Input: part model. Units: mm. Frame: model coordinates. A direction names the side the tool comes from. Round coordinates to 2 decimals unless told otherwise and drop trailing zeros. Order: outer loops, then holes, each group sorted by start corner. A loop starts at its lowest first (then second) coordinate and runs counter-clockwise, first axis right, second up. Notation, with made-up numbers: (56, 86) - (113, 86) arc R21 ccw to (113, 120) - close; hole circle Ø5 at (38.5, 10.5). An arc over 180 degrees is marked (long way). One line per item, written item: value. Start each with the question number.
from build123d import *

# Parameters (mm, degrees)
BOSS_EXTRUDE6_DEPTH  = 2.05994
SKETCH9_W            = 27.13228
SKETCH9_H            = 1.41224
BOSS_EXTRUDE7_DEPTH  = 20.32
SKETCH10_R           = 2.50063
CUT_EXTRUDE3_DEPTH   = 25.4
BOSS_EXTRUDE10_DEPTH = 16.02994
SKETCH15_W           = 51.72964
SKETCH15_H           = 37.846
CUT_EXTRUDE5_DEPTH   = 64.999044225
SKETCH16_W           = 27.13228
SKETCH16_H           = 1.41224
BOSS_EXTRUDE11_DEPTH = 3.175
SKETCH18_W           = 12.7
SKETCH18_H           = 2.54
BOSS_EXTRUDE12_DEPTH = 12.7
SKETCH19_R           = 2.159
CUT_EXTRUDE6_DEPTH   = 62.075806811


with BuildPart() as part:
    # Sketch8 → Boss-Extrude6 (new body)
    with BuildSketch(Plane(origin=(0, 0, 0), x_dir=(1, 0, 0), z_dir=(0, 1, 0))):
        Polygon((-44.974060072, -2.900891689), (-44.974060072, -40.746891689), (2.165799928, -40.746891689), (2.165799928, -35.808024144), (6.755579928, -31.218244144), (33.887859928, -31.218244144), (33.887859928, -12.429539234), (6.755579928, -12.429539234), (2.165799928, -7.839759234), (2.165799928, -2.900891689), align=None)
    extrude(amount=BOSS_EXTRUDE6_DEPTH)

    # Sketch9 → Boss-Extrude7 (add)
    with BuildSketch(Plane(origin=(0, 2.05994, 0), x_dir=(1, 0, 0), z_dir=(0, 1, 0))):
        with Locations((20.321719928, -13.135659234)):
            Rectangle(SKETCH9_W, SKETCH9_H)
        with Locations((20.321719928, -30.512124144)):
            Rectangle(SKETCH9_W, SKETCH9_H)
    extrude(amount=BOSS_EXTRUDE7_DEPTH)

    # Sketch10 → Cut-Extrude3 (cut)
    with BuildSketch(Plane.XY.offset(31.218244144)):
        with Locations((29.955939928, 17.2847)):
            Circle(SKETCH10_R)
    extrude(amount=-CUT_EXTRUDE3_DEPTH, mode=Mode.SUBTRACT)

    # Sketch14 → Boss-Extrude10 (add)
    with BuildSketch(Plane.XY.offset(13.841779234)):
        Polygon((6.755579928, 22.37994), (33.887859928, 2.05994), (30.568919609, 2.05994), (6.755579928, 19.826826768), align=None)
    extrude(amount=BOSS_EXTRUDE10_DEPTH)

    # Sketch15 → Cut-Extrude5 (cut, through all)
    with BuildSketch(Plane(origin=(0, 2.05994, 0), x_dir=(1, 0, 0), z_dir=(0, 1, 0))):
        with Locations((-19.109240072, -21.823891689)):
            Rectangle(SKETCH15_W, SKETCH15_H)
    extrude(amount=-CUT_EXTRUDE5_DEPTH, mode=Mode.SUBTRACT)

    # Sketch16 → Boss-Extrude11 (add)
    with BuildSketch(Plane(origin=(0, 22.37994, 0), x_dir=(1, 0, 0), z_dir=(0, 1, 0))):
        with Locations((20.321719928, -30.512124144)):
            Rectangle(SKETCH16_W, SKETCH16_H)
        with Locations((20.321719928, -13.135659234)):
            Rectangle(SKETCH16_W, SKETCH16_H)
    extrude(amount=BOSS_EXTRUDE11_DEPTH)

    # Sketch18 → Boss-Extrude12 (add)
    with BuildSketch(Plane.XY.offset(31.218244144)):
        with Locations((13.105579928, 24.28494)):
            Rectangle(SKETCH18_W, SKETCH18_H)
    boss_extrude12 = extrude(amount=BOSS_EXTRUDE12_DEPTH)

    # Mirror1: Boss-Extrude12 across plane
    add(boss_extrude12.mirror(Plane.XY.offset(21.823891689)))

    # Sketch19 → Cut-Extrude6 (cut, through all)
    with BuildSketch(Plane(origin=(0, 25.55494, 0), x_dir=(1, 0, 0), z_dir=(0, 1, 0))):
        with Locations(Location((13.105579928, -6.079539234, 0), (0, 0, 270))):
            Circle(SKETCH19_R)
        with Locations(Location((13.105579928, -37.568244144, 0), (0, 0, 270))):
            Circle(SKETCH19_R)
    extrude(amount=-CUT_EXTRUDE6_DEPTH, mode=Mode.SUBTRACT)


solid = part.part
1. Section B-B (x = 20.5). Return the cut outline in (y, z), then the cut area to 3 significant figures.
2. Section D-D (y = 10.5). Return the cut outline in (x, z).
3. Set-up query: faces 1 (the face through (16, 23.015, 6)), 2 (the face through (18, 2.06, 22)), 3 (the face through (19.456, 24, 37)), 4 (the face through (23, 19, 29.806)), 5 (the face through (13, 24, 43.918)). Return all of +Z, -Z, +X, -X, +Y, -Y with unobstructed straight access to the full face (end or side cutting, diameter ignored); none if empty.
4. Section A-A (x = 14.25). Return the cut outline in (y, z).
5. Pin query (flat end, axial travel): pin 1 (11.5 mm diameter, centred on x = 20, y = 15, fed in from -Z); pin 2 (7.5 mm diameter, centred on x = 18.5, y = 6.5, fed in from +Z); pin 3 (6.5 mm diameter, centred on x = 14.5, z = 7.5, fed in from -Y); pin 4 (4.5 mm diameter, centred on x = 29.96, y = 17.28, fed in from -Z). Return the tip coordinate at first contact, or that it passes through.
6. Line query: line 1 (Z direction, x = 20.75, y = 22); line 2 (Z direction, x = 12.5, y = 24.5); line 3 (Y direction, x = 14.25, z = 27). Output: solid intervals per line, ascending. Write a range as from..to.
7. Section C-C (z = 7). Return the cut outline in (x, y), then the cut area to 3 significant figures.
8. Pull-direction query (X, two-part tool) for faces 6 (the face through (15.246, 24.303, 5.798)), 7 (the face through (13, 23.015, 40)), 8 (the face through (19.456, 24, 6)), 9 (the face through (27.458, 17.395, 30.522)); classes: released by +X, released by -X, zero draft, split by the parting line, or undercut.
Solved:
1. outline: (0, 12.43) - (25.55, 12.43) - (25.55, 13.84) - (12.09, 13.84) - (12.09, 29.81) - (25.55, 29.81) - (25.55, 31.22) - (0, 31.22) - close; hole (2.06, 13.84) - (9.57, 13.84) - (9.57, 29.81) - (2.06, 29.81) - close
1. area: 145 mm²
2. outline: (6.76, 12.43) - (33.89, 12.43) - (33.89, 13.84) - (22.62, 13.84) - (22.62, 29.81) - (33.89, 29.81) - (33.89, 31.22) - (6.76, 31.22) - (6.76, 29.81) - (19.26, 29.81) - (19.26, 13.84) - (6.76, 13.84) - close
3. face 1: -Z, +X, -X, -Y
3. face 2: -X
3. face 3: +Z, +X, +Y, -Y
3. face 4: +X, +Y
3. face 5: +Z, +X, -X, +Y, -Y
4. outline: (0, 12.43) - (23.01, 12.43) - (23.01, 7.91) - (25.55, 7.91) - (25.55, 13.84) - (16.77, 13.84) - (16.77, 29.81) - (25.55, 29.81) - (25.55, 35.74) - (23.01, 35.74) - (23.01, 31.22) - (0, 31.22) - close; (23.01, -0.27) - (25.55, -0.27) - (25.55, 4.25) - (23.01, 4.25) - close; (23.01, 39.4) - (25.55, 39.4) - (25.55, 43.92) - (23.01, 43.92) - close; hole (2.06, 13.84) - (14.24, 13.84) - (14.24, 29.81) - (2.06, 29.81) - close
5. pin 1: stops at z = 12.43
5. pin 2: stops at z = 31.22
5. pin 3: stops at y = 23.01
5. pin 4: passes through
6. line 1: z = 12.43..13.84, 29.81..31.22
6. line 2: z = -0.27..4.01, 8.15..13.84, 29.81..35.5, 39.64..43.92
6. line 3: y = 0..2.06, 14.24..16.77
7. outline: (6.76, 23.01) - (11.15, 23.01) - (11.15, 25.55) - (6.76, 25.55) - close; (15.06, 23.01) - (19.46, 23.01) - (19.46, 25.55) - (15.06, 25.55) - close
7. area: 22.3 mm²
8. face 6: undercut
8. face 7: zero draft
8. face 8: released by +X
8. face 9: undercut
